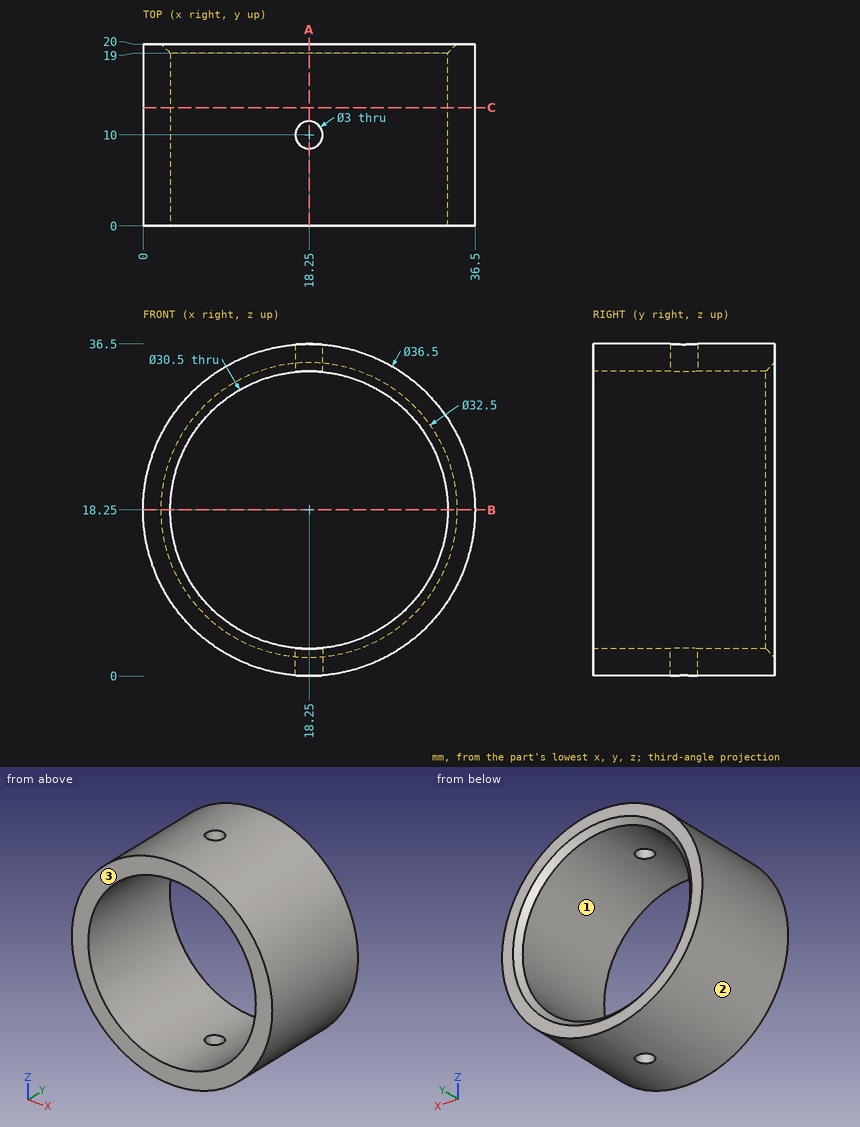
For this review, use the dimensioned drawing (mm, ordinates from the lowest corner) and the shaded views. Coordinates: 2 decimals unless noted, no trailing zeros. Loops run counter-clockwise (first coordinate to the right, second up) from the corner with the lowest first, then second, coordinate; pieces in that order, holes last.
1. Mouldability with a two-part tool opening along X and no side actions: class the marked faces 1, 2 and 3 as +X half, -X half, draft (parallel to the pull), parting line (faces both ways), or undercut.
2. For line 1 (Z direction, x = 18.25, y = 4.25); line 2 (Y direction, x = 18.25, z = 35.6); line 3 (X direction, y = 5.5, z = 31.5), list the stretches that pass through material, from the lowest coordinate up.
3. Insertion check: P1, Ø6, axis at y = 10, z = 22, coming from the -X side; P2, Ø1.5, axis at y = 4.5, z = 22.5, coming from the +X side; P3, Ø2.5, axis at x = 18.25, y = 10, coming from the +Z side; P4, Ø10, axis at x = 22, y = 6.5, coming from the -Z side. Each pin has a flat end and moves straight along its axis. Give the tip position at first contact, or say it passes through.
4. Add section A-A, the plane x = 18.25. Give the boundary of the cut face in (y, z), then the cut area to 3 significant figures.
5. Add section B-B, the plane z = 18.25. Give the boundary of the cut face in (x, y), then the cut area to 3 significant figures.
6. Add section C-C, the plane y = 13. Give the boundary of the cut face in (x, z).
Result:
1. face 1: undercut
1. face 2: parting line
1. face 3: draft
2. line 1: z = 0 to 3, 33.5 to 36.5
2. line 2: y = 0 to 8.5, 11.5 to 20
2. line 3: x = 5.7 to 10.7, 25.8 to 30.8
3. P1: stops at x = 0.02
3. P2: stops at x = 36.16
3. P3: passes through
3. P4: stops at z = 0
4. outline: (0, 0) - (8.5, 0) - (8.5, 3) - (0, 3) - close; (0, 33.5) - (8.5, 33.5) - (8.5, 36.5) - (0, 36.5) - close; (11.5, 0) - (20, 0) - (20, 2) - (19, 3) - (11.5, 3) - close; (11.5, 33.5) - (19, 33.5) - (20, 34.5) - (20, 36.5) - (11.5, 36.5) - close
4. area: 101 mm2
5. outline: (0, 0) - (3, 0) - (3, 19) - (2, 20) - (0, 20) - close; (33.5, 0) - (36.5, 0) - (36.5, 20) - (34.5, 20) - (33.5, 19) - close
5. area: 119 mm2
6. outline: circle Ø36.5 at (18.25, 18.25); hole circle Ø30.5 at (18.25, 18.25)
